Verification items for this drawing (mm, ordinates from the low corner). A direction names the side the tool comes from. Give positions to 0.01 mm unless a question says otherwise; leave off trailing zeros. Order: outer loops, then holes, each group sorted by start corner. A loop starts at its lowest first (then second) coordinate and runs counter-clockwise, first axis right, second up. Notation, with made-up numbers: (85.25, -5.5) -> (118.25, -5.5) arc R21 cw to (118.25, 26.5) -> close; hole circle Ø5 at (-25.5, 89). An arc over 180 degrees is marked (long way). One line per question, with ' | ' between items.
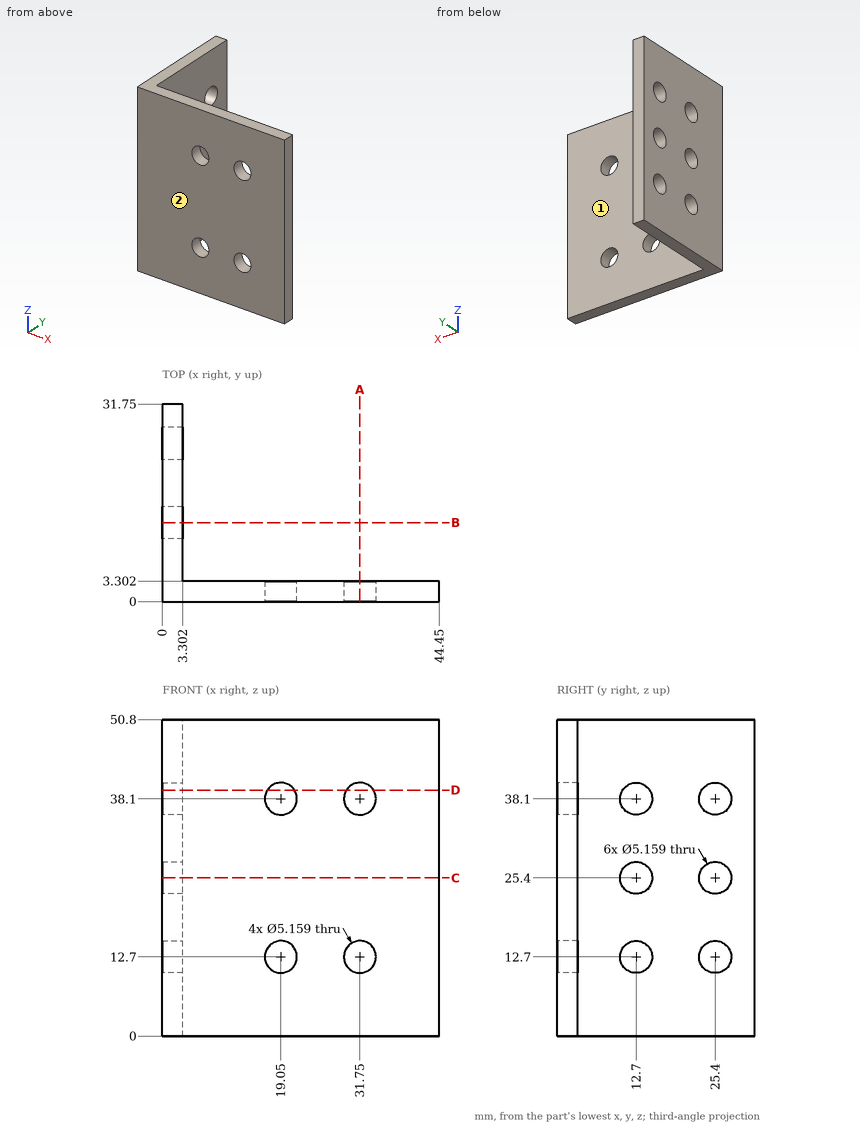
Q1. Section check B-B (y = 12.7). Enter the section's corners in (x, z).
Result sheet:
outline: (0, 0) -> (3.3, 0) -> (3.3, 10.12) -> (0, 10.12) -> close; (0, 15.28) -> (3.3, 15.28) -> (3.3, 22.82) -> (0, 22.82) -> close; (0, 27.98) -> (3.3, 27.98) -> (3.3, 35.52) -> (0, 35.52) -> close; (0, 40.68) -> (3.3, 40.68) -> (3.3, 50.8) -> (0, 50.8) -> close
Q2. Section check D-D (z = 39.5). Enter the section's corners in (x, y).
Result sheet:
outline: (0, 0) -> (16.88, 0) -> (16.88, 3.3) -> (3.3, 3.3) -> (3.3, 10.53) -> (0, 10.53) -> close; (0, 14.87) -> (3.3, 14.87) -> (3.3, 23.23) -> (0, 23.23) -> close; (0, 27.57) -> (3.3, 27.57) -> (3.3, 31.75) -> (0, 31.75) -> close; (21.22, 0) -> (29.58, 0) -> (29.58, 3.3) -> (21.22, 3.3) -> close; (33.92, 0) -> (44.45, 0) -> (44.45, 3.3) -> (33.92, 3.3) -> close
Q3. Thickness scan on line 1 (Z direction, x = 31.75, y = 2); line 2 (X direction, y = 2, z = 38); line 3 (Y direction, x = 2.35, z = 12.7). Record the ranges inside material, lowest first.
Result sheet:
line 1: z = 0 to 10.12, 15.28 to 35.52, 40.68 to 50.8 | line 2: x = 0 to 16.47, 21.63 to 29.17, 34.33 to 44.45 | line 3: y = 0 to 10.12, 15.28 to 22.82, 27.98 to 31.75
Q4. Access from +Z, -Z, +X, -X, +Y, -Y to the whole of each face (thin tool, end or side, straight path). Record for the marked faces 1 and 2.
Result sheet:
face 1: +Z, -Z, +X, +Y | face 2: +Z, -Z, +X, -X, -Y
Q5. Depth check by flat-ended pin: pin 1 Ø1 at (y, z) = (7.5, 44.5) entering from +X; pin 2 Ø6 at (x, z) = (19.05, 38.1) entering from +Y. Enter the tip coordinate at first touch or a pass-through.
Result sheet:
pin 1: stops at x = 3.3 | pin 2: stops at y = 3.3
Q6. Section check C-C (z = 25.4). Enter the section's corners in (x, y).
Result sheet:
outline: (0, 0) -> (44.45, 0) -> (44.45, 3.3) -> (3.3, 3.3) -> (3.3, 10.12) -> (0, 10.12) -> close; (0, 15.28) -> (3.3, 15.28) -> (3.3, 22.82) -> (0, 22.82) -> close; (0, 27.98) -> (3.3, 27.98) -> (3.3, 31.75) -> (0, 31.75) -> close
Q7. Section check A-A (x = 31.75). Enter the section's corners in (y, z).
Result sheet:
outline: (0, 0) -> (3.3, 0) -> (3.3, 10.12) -> (0, 10.12) -> close; (0, 15.28) -> (3.3, 15.28) -> (3.3, 35.52) -> (0, 35.52) -> close; (0, 40.68) -> (3.3, 40.68) -> (3.3, 50.8) -> (0, 50.8) -> close
